```python
from build123d import *

# Parameters (mm, degrees)
F0_R     = 9
F1_DEPTH = 4
F2_W     = 3
F2_H     = 3
F3_DEPTH = 2
F5_R     = 9
F5_R_2   = 8
F5_W     = 0.3704614937
F5_H     = 1.2024026364
F4_DEPTH = 1


with BuildPart() as f1:
    # F0 (on Top) → F1 (new body)
    with BuildSketch(Plane.XY):
        with Locations((-31.3306450844, 19.7580661625)):
            Circle(F0_R)
    extrude(amount=F1_DEPTH)

    # F2 (on face) → F3 (cut)
    with BuildSketch(Plane(origin=(0, 0, 0), x_dir=(1, 0, 0), z_dir=(0, 0, -1))):
        with BuildLine():
            ThreePointArc((-32.8306450844, -28.6321858371), (-32.0832814269, -28.7265408676), (-31.3306450844, -28.7580661625))
            ThreePointArc((-31.3306450844, -28.7580661625), (-30.5780087419, -28.7265408676), (-29.8306450844, -28.6321858371))
            Line((-29.8306450844, -28.6321858371), (-29.8306450844, -21.2580661625))
            Line((-29.8306450844, -21.2580661625), (-32.8306450844, -21.2580661625))
            Line((-32.8306450844, -21.2580661625), (-32.8306450844, -28.6321858371))
        make_face()
        with BuildLine():
            ThreePointArc((-40.204764759, -18.2580661625), (-40.2991197895, -19.0054298199), (-40.3306450844, -19.7580661625))
            ThreePointArc((-40.3306450844, -19.7580661625), (-40.2991197895, -20.510702505), (-40.204764759, -21.2580661625))
            Line((-40.204764759, -21.2580661625), (-32.8306450844, -21.2580661625))
            Line((-32.8306450844, -21.2580661625), (-32.8306450844, -18.2580661625))
            Line((-32.8306450844, -18.2580661625), (-40.204764759, -18.2580661625))
        make_face()
        with Locations((-31.3306450844, -19.7580661625)):
            Rectangle(F2_W, F2_H)
        with BuildLine():
            Line((-29.8306450844, -18.2580661625), (-29.8306450844, -21.2580661625))
            Line((-29.8306450844, -21.2580661625), (-22.4565254097, -21.2580661625))
            ThreePointArc((-22.4565254097, -21.2580661625), (-22.3621703793, -20.510702505), (-22.3306450844, -19.7580661625))
            ThreePointArc((-22.3306450844, -19.7580661625), (-22.3621703793, -19.0054298199), (-22.4565254097, -18.2580661625))
            Line((-22.4565254097, -18.2580661625), (-29.8306450844, -18.2580661625))
        make_face()
        with BuildLine():
            Line((-32.8306450844, -10.8839464878), (-32.8306450844, -18.2580661625))
            Line((-32.8306450844, -18.2580661625), (-29.8306450844, -18.2580661625))
            Line((-29.8306450844, -18.2580661625), (-29.8306450844, -10.8839464878))
            ThreePointArc((-29.8306450844, -10.8839464878), (-30.5780087419, -10.7895914574), (-31.3306450844, -10.7580661625))
            ThreePointArc((-31.3306450844, -10.7580661625), (-32.0832814269, -10.7895914574), (-32.8306450844, -10.8839464878))
        make_face()
    extrude(amount=-F3_DEPTH, mode=Mode.SUBTRACT)

    # F5 (on face) → F4 (join)
    with BuildSketch(Plane.XY.offset(4)):
        with Locations((-31.3306450844, 19.7580661625)):
            Circle(F5_R)
        with Locations((-31.3306450844, 19.7580661625)):
            Circle(F5_R_2, mode=Mode.SUBTRACT)
        Polygon((-33.3540178835, 24.8932279646), (-36.2118817866, 24.328712374), (-35.2945402265, 23.0938345194), (-35.929620266, 19.1775020212), (-36.4941395819, 17.6956485957), (-37.51732409, 17.4133908004), (-37.51732409, 16.5313333273), (-36.8822440505, 16.0726644099), (-36.0354706645, 16.4960511029), (-35.1886935532, 18.4365753084), (-33.4951467812, 18.4365753084), (-33.4951467812, 18.7893975526), (-27.5677256286, 18.7893975526), (-28.5203475505, 16.4607688785), (-32.7542200685, 16.4607688785), (-30.7431295514, 15.0141958147), (-27.885267511, 15.0141958147), (-26.2270011008, 19.0010908991), (-25.4155080765, 20.3065350652), (-30.5314362049, 20.3065350652), (-30.5314362049, 20.9768973291), (-27.4618789554, 20.9768973291), (-27.0737744868, 21.6119792312), (-30.4608717561, 21.6119792312), (-30.4608717561, 22.0000836998), (-27.0032100379, 22.0000836998), (-26.6856700182, 23.0232700706), (-30.3903073072, 23.0232700706), (-30.3903073072, 23.7994790077), (-26.4739766717, 23.7994790077), (-26.756234467, 24.8932279646), align=None)
        Polygon((-34.499656409, 19.8707804084), (-34.7300246358, 20.377099514), (-34.2007912695, 20.6392026472), (-31.7267395564, 20.6392026472), (-31.6514596343, 20.258097545), (-32.6876805022, 20.258097545), (-33.209066838, 19.8707804084), align=None, mode=Mode.SUBTRACT)
        Polygon((-34.2753518545, 21.7523517899), (-33.7431058288, 22.3036166281), (-31.5476171672, 22.3036166281), (-31.5476171672, 21.7250771821), (-33.0903939903, 21.7250771821), (-33.5618001374, 21.3748883364), (-34.2007912695, 21.3748883364), align=None, mode=Mode.SUBTRACT)
        Polygon((-34.3772023916, 23.058552295), (-34.2007912695, 23.3408100903), (-33.7020926227, 23.7112734467), (-31.5899029374, 23.7112734467), (-31.6957496107, 23.058552295), align=None, mode=Mode.SUBTRACT)
        Polygon((-33.7434709072, 17.5698362291), (-34.3099012971, 17.5698362291), (-34.3099012971, 17.234172672), (-33.4497652948, 17.234172672), (-33.4497652948, 17.9789252579), (-33.7434709072, 17.9789252579), align=None)
        with Locations((-31.9214742631, 17.8353739902)):
            Rectangle(F5_W, F5_H)
        Polygon((-29.3105877936, 18.5256265104), (-30.2191060036, 18.5256265104), (-30.2191060036, 18.1992650032), (-29.707511887, 18.1992650032), (-29.707511887, 17.784697935), (-29.2753055692, 17.784697935), (-29.2753055692, 17.234172672), (-28.9842262864, 17.234172672), (-28.9842262864, 18.0316753685), (-29.3105877936, 18.0316753685), align=None)
    extrude(amount=F4_DEPTH)


solid = f1.part
```
Here's how the part is built. I have some questions about the finished solid (model axes, mm). A direction names the side the tool comes from. Round coordinates to 2 decimals unless told otherwise and drop trailing zeros. Write each loop counter-clockwise with the first axis right and the second up, starting at its lowest first coordinate (ties: lowest second). Pieces come first, ordered by that corner, then holes.
Q1. If we section it at B-B on x = -24.75: Write out the boundary of the cut face in (y, z), plus the area to 3 significant figures.
Q2. Will these pins go through, and if not, where does the flat tip stop? P1, Ø1, axis at x = -26.5, z = 1.5, coming from the +Y side; P2, Ø2, axis at y = 15.5, z = 1.5, coming from the -X side; P3, Ø0.5, axis at y = 18, z = 4.5, coming from the +X side.
Q3. If we section it at C-C on y = 17: Write out the boundary of the cut face in (x, z), plus the area to 3 significant figures.
Q4. If we section it at D-D on y = 26.75: Write out the boundary of the cut face in (x, z).
Q5. If we mould it in two halves opening along Y, with no side actions, what happens to faces 5 (the cylindrical face through (-27.178, 11.774, 2.465)), 6 (the flat face through (-32.7, 22.304, 4.5)), 7 (the flat face through (-32, 20, 5))? For each: +Y half, -Y half, draft (parallel to the pull), parting line (faces both ways), or undercut.
Q6. Which directions (+Z, -Z, +X, -X, +Y, -Y) give clear straight access to the entire face, cutting with the end or side of a thin tool? Please do faces 1 (the flat face through (-33.8, 19.871, 4.5)), 2 (the flat face through (-27, 24, 0)), 3 (the flat face through (-32.831, 15, 1)), 4 (the flat face through (-26, 18.258, 1)).
Q7. Please list where these lines run through material, in increasing order: probe 1 along X at (y, z) = (21.5, 4.3); probe 2 along Z at (x, y) = (-32.25, 12.75); probe 3 along Z at (x, y) = (-33.5, 25.75).
Q8. If we section it at A-A on z = 0.6: Write out the boundary of the cut face in (x, y), plus the area to 3 significant figures.
Answer below:
1. outline: (13.62, 0) - (18.26, 0) - (18.26, 2) - (21.26, 2) - (21.26, 0) - (25.9, 0) - (25.9, 5) - (24.31, 5) - (24.31, 4) - (15.21, 4) - (15.21, 5) - (13.62, 5) - close
1. area: 46.3 mm2
2. P1: stops at y = 27.65
2. P2: stops at x = -39.72
2. P3: stops at x = -22.46
3. outline: (-39.9, 0) - (-32.83, 0) - (-32.83, 2) - (-29.83, 2) - (-29.83, 0) - (-22.76, 0) - (-22.76, 5) - (-23.82, 5) - (-23.82, 4) - (-27.06, 4) - (-27.06, 5) - (-28.3, 5) - (-28.3, 4) - (-35.82, 4) - (-35.82, 5) - (-37.52, 5) - (-37.52, 4) - (-38.84, 4) - (-38.84, 5) - (-39.9, 5) - close
3. area: 67.6 mm2
4. outline: (-37, 0) - (-32.83, 0) - (-32.83, 2) - (-29.83, 2) - (-29.83, 0) - (-25.66, 0) - (-25.66, 5) - (-27.44, 5) - (-27.44, 4) - (-35.22, 4) - (-35.22, 5) - (-37, 5) - close
5. face 5: parting line
5. face 6: undercut
5. face 7: draft
6. face 1: +Z
6. face 2: -Z, +X, -X, +Y, -Y
6. face 3: -Z, +Y, -Y
6. face 4: -Z, +X, -X
7. probe 1: x = -40.16 to -39.14, -35.55 to -34.23, -33.39 to -27.14, -23.52 to -22.5
7. probe 2: z = 2 to 4
7. probe 3: z = 0 to 4
8. outline: (-40.2, 18.26) arc R9 ccw to (-32.83, 10.88) - (-32.83, 18.26) - close; (-40.2, 21.26) - (-32.83, 21.26) - (-32.83, 28.63) arc R9 ccw to start; (-29.83, 10.88) arc R9 ccw to (-22.46, 18.26) - (-29.83, 18.26) - close; (-29.83, 21.26) - (-22.46, 21.26) arc R9 ccw to (-29.83, 28.63) - close
8. area: 156 mm2
